```python
from build123d import *

# Parameters (mm, degrees)
F0_W     = 40
F0_H     = 46
F1_DEPTH = 40
F2_R     = 18
F3_DEPTH = 26
F4_R     = 18
F5_DEPTH = 26
F8_D     = 18
F6_W     = 24
F6_H     = 30
F9_DEPTH = 50


with BuildPart() as f1:
    # F0 (on Top) → F1 (new body)
    with BuildSketch(Plane.XY):
        with Locations((-54.399494, -49.857425)):
            Rectangle(F0_W, F0_H)
    extrude(amount=F1_DEPTH)

    # F2 (on face) → F3 (join)
    with BuildSketch(Plane.XZ.offset(72.857425)):
        with Locations((-54.399494, 20)):
            Circle(F2_R)
    extrude(amount=F3_DEPTH)

    # F4 (on face) → F5 (join)
    with BuildSketch(Plane(origin=(0, -26.857425, 0), x_dir=(-1, 0, 0), z_dir=(0, 1, 0))):
        with Locations((54.399494, 20)):
            Circle(F4_R)
    extrude(amount=F5_DEPTH)

    # F8 (through all)
    with Locations(Plane(origin=(0, -0.857425, 0), x_dir=(-1, 0, 0), z_dir=(0, 1, 0))):
        with Locations((54.399494, 20)):
            Hole(F8_D / 2)

    # F6 (on face) → F9 (cut)
    with BuildSketch(Plane(origin=(-74.399494, 0, 0), x_dir=(0, -1, 0), z_dir=(-1, 0, 0))):
        with Locations((49.857425, 20)):
            Rectangle(F6_W, F6_H)
    extrude(amount=-F9_DEPTH, mode=Mode.SUBTRACT)


solid = f1.part
```
Build history of the part. All positions in model axes, mm. A direction names the side the tool comes from. Round coordinates to 2 decimals unless told otherwise and drop trailing zeros. Loops run counter-clockwise (first coordinate to the right, second up) from the corner with the lowest first, then second, coordinate; pieces in that order, holes last.
Item 1: Pin check, flat tips, straight feed: P1, Ø12, axis at y = -86, z = 15.5, coming from the -X side; P2, Ø3, axis at x = -52, y = -82.5, coming from the +Z side; P3, Ø4, axis at x = -61, y = -19.5, coming from the +Z side. Stop position of each tip, or through.
Item 2: Saw through at A-A (z = 20). List the corners of the cut face in (x, y), then the cut area to 3 significant figures.
Item 3: Saw through at B-B (y = -40). List the corners of the cut face in (x, z), then the cut area to 3 significant figures.
Item 4: Drill centre lines: line 1 along Z through (x, y) = (-53, -39); line 2 along Y through (x, z) = (-40.5, 14); line 3 along Z through (x, y) = (-54, -7). Where is each one in solid material? Low to high.
Item 5: Which spindle directions (+Z, -Z, +X, -X, +Y, -Y) get a long thin tool onto all of the face, cutting with end or side? Do faces 4 (the face through (-46, -0.857, 16)), 5 (the face through (-40.115, -14.039, 9.047)), 6 (the face through (-72, -72.857, 15)), 7 (the face through (-64, -37.857, 20)), 8 (the face through (-55.571, -19.616, 28.923)). Say none if no direction does.
Item 6: Two-plate mould, pull along Y, no slides. Class faces 1 (the face through (-55, -50, 0)), 2 (the face through (-72, -26.857, 15)), 3 (the face through (-55, -50, 35)): released by +Y, released by -Y, zero draft, split by the parting line, or undercut.
Item 7: Saw through at D-D (x = -59). List the corners of the cut face in (y, z), then the cut area to 4 significant figures.
Item 8: Saw through at C-C (x = -70). List the corners of the cut face in (y, z).
Worked answers:
1. P1: stops at x = -72.4
1. P2: stops at z = 37.98
1. P3: stops at z = 37.4
2. outline: (-74.4, -72.86) - (-72.4, -72.86) - (-72.4, -98.86) - (-63.4, -98.86) - (-63.4, -61.86) - (-74.4, -61.86) - close; (-74.4, -37.86) - (-63.4, -37.86) - (-63.4, -0.86) - (-72.4, -0.86) - (-72.4, -26.86) - (-74.4, -26.86) - close; (-45.4, -98.86) - (-36.4, -98.86) - (-36.4, -72.86) - (-34.4, -72.86) - (-34.4, -61.86) - (-45.4, -61.86) - close; (-45.4, -37.86) - (-34.4, -37.86) - (-34.4, -26.86) - (-36.4, -26.86) - (-36.4, -0.86) - (-45.4, -0.86) - close
2. area: 1,420 mm2
3. outline: (-74.4, 0) - (-34.4, 0) - (-34.4, 5) - (-74.4, 5) - close; (-74.4, 35) - (-34.4, 35) - (-34.4, 40) - (-74.4, 40) - close
3. area: 400 mm2
4. line 1: z = 0 to 5, 35 to 40
4. line 2: y = -98.86 to -61.86, -37.86 to -0.86
4. line 3: z = 2 to 11.01, 28.99 to 38
5. face 4: +Z, -Z, +X, -X, +Y
5. face 5: +Y
5. face 6: -Y
5. face 7: +X, -X
5. face 8: +Y, -Y
6. face 1: zero draft
6. face 2: released by +Y
6. face 3: undercut
7. outline: (-98.86, 2.6) - (-72.86, 2.6) - (-72.86, 0) - (-26.86, 0) - (-26.86, 2.6) - (-0.86, 2.6) - (-0.86, 12.26) - (-37.86, 12.26) - (-37.86, 5) - (-61.86, 5) - (-61.86, 12.26) - (-98.86, 12.26) - close; (-98.86, 27.74) - (-61.86, 27.74) - (-61.86, 35) - (-37.86, 35) - (-37.86, 27.74) - (-0.86, 27.74) - (-0.86, 37.4) - (-26.86, 37.4) - (-26.86, 40) - (-72.86, 40) - (-72.86, 37.4) - (-98.86, 37.4) - close
7. area: 1,785 mm2
8. outline: (-98.86, 11.02) - (-72.86, 11.02) - (-72.86, 0) - (-26.86, 0) - (-26.86, 11.02) - (-0.86, 11.02) - (-0.86, 28.98) - (-26.86, 28.98) - (-26.86, 40) - (-72.86, 40) - (-72.86, 28.98) - (-98.86, 28.98) - close; hole (-61.86, 5) - (-37.86, 5) - (-37.86, 35) - (-61.86, 35) - close
